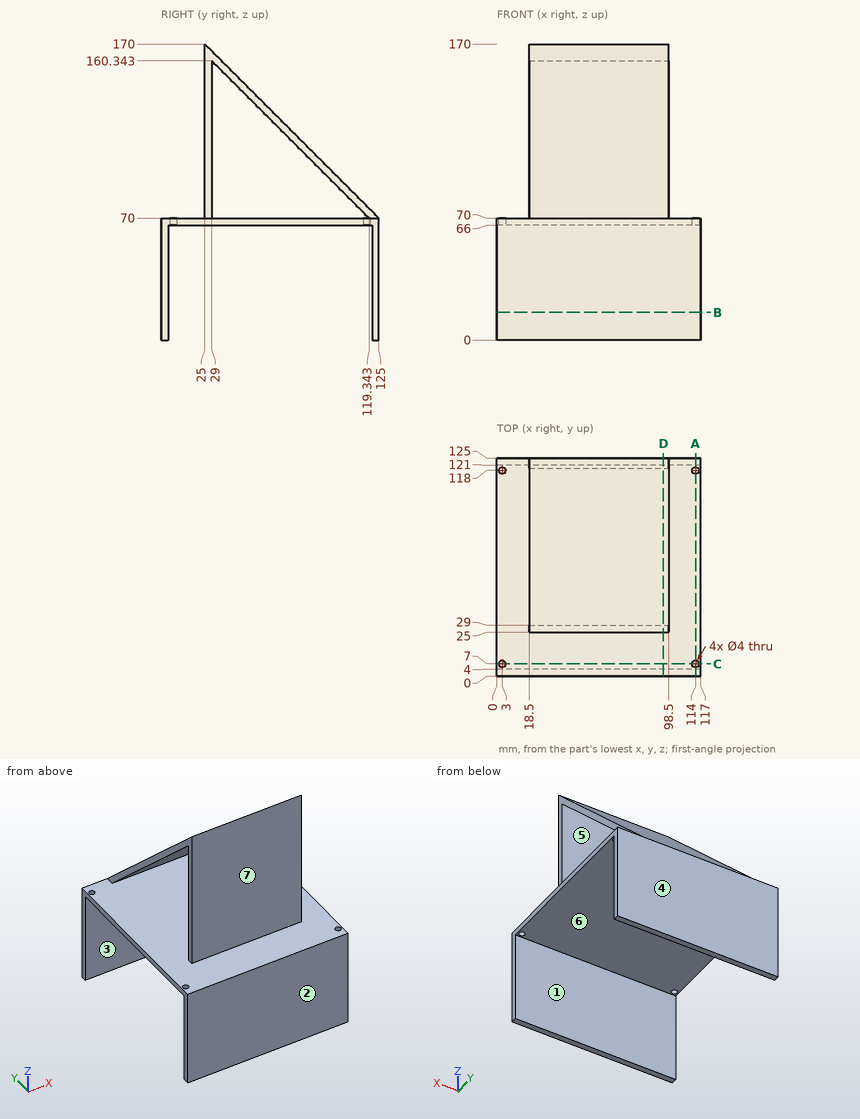
Could you check a few things on this drawing? It's one solid part, dimensions in mm from its lowest x, y, z. A direction names the side the tool comes from. Give positions to 0.01 mm unless a question says otherwise; leave off trailing zeros. Order: outer loops, then holes, each group sorted by start corner. A loop starts at its lowest first (then second) coordinate and runs counter-clockwise, first axis right, second up. Notation, with made-up numbers: M 25,65.5 L 69,65.5 A36 ccw 69,104.5 Z; hole C 74,-27 d2. An arc over 180 degrees is marked long. Use one line per item in the form item = value.
Item 1: If we section it at B-B, the plane z = 16: Write out the boundary of the cut face in (x, y), and give its area (3 significant figures).
Values follow:
outline = M 0,0 L 117,0 L 117,4 L 0,4 Z; M 0,121 L 117,121 L 117,125 L 0,125 Z
area = 936 mm^2
Item 2: If we section it at A-A, the plane x = 114: Write out the boundary of the cut face in (y, z), and give its area (3 significant figures).
Values follow:
outline = M 0,0 L 4,0 L 4,66 L 5,66 L 5,70 L 0,70 Z; M 9,66 L 116,66 L 116,70 L 9,70 Z; M 120,66 L 121,66 L 121,0 L 125,0 L 125,70 L 120,70 Z
area = 996 mm^2
Item 3: For the marked faces 5, 6 and 7, which set-ups out of +Z, -Z, +X, -X, +Y, -Y let a thin tool reach every point of the face, with its end or its side?
Values follow:
face_5 = +X, -X
face_6 = -Z, +X, -X
face_7 = +Z, +X, -X, -Y
Item 4: If we section it at D-D, the plane x = 95.5: Write out the boundary of the cut face in (y, z).
Values follow:
outline = M 0,0 L 4,0 L 4,66 L 121,66 L 121,0 L 125,0 L 125,70 L 25,170 L 25,70 L 0,70 Z; hole M 29,70 L 119.34,70 L 29,160.34 Z
Item 5: If I drill on line 1 along Y through (x, z) = (3, 69.1); line 2 along Y through (x, z) = (31.5, 45); line 3 along Z through (x, y) = (9, 51.5), over which ranges is the centre line in solid material (lowest first)? Write a range as [from, to].
Values follow:
line_1 = [0, 5], [9, 116], [120, 125]
line_2 = [0, 4], [121, 125]
line_3 = [66, 70]
Item 6: If we section it at C-C, the plane y = 7: Write out the boundary of the cut face in (x, z).
Values follow:
outline = M 0,66 L 1,66 L 1,70 L 0,70 Z; M 5,66 L 112,66 L 112,70 L 5,70 Z; M 116,66 L 117,66 L 117,70 L 116,70 Z
Item 7: Will these pins go through, and if not, where does the flat tip stop? pin 1 Ø4 at (x, y) = (23.5, 67) entering from +Z; pin 2 Ø3 at (x, y) = (85, 23) entering from -Z; pin 3 Ø20 at (x, z) = (31, 36) entering from -Y; pin 4 Ø5 at (x, y) = (41.5, 29.5) entering from +Z.
Values follow:
pin_1 = 130
pin_2 = 66
pin_3 = 0
pin_4 = 168
Item 8: Thinking about a two-plate mould opening in Y: for the marked faces 1, 2, 3 and 4, which applies, pulls with the +Y half, pulls with the -Y half, needs draft (parallel to the pull), parting line crosses it, or undercut?
Values follow:
face_1 = undercut
face_2 = pulls with the -Y half
face_3 = undercut
face_4 = pulls with the +Y half
